The model under review builds one solid part; all positions refer to its coordinate system, in mm. A direction names the side the tool comes from. Coordinates: 2 decimals unless noted, no trailing zeros. Loops run counter-clockwise (first coordinate to the right, second up) from the corner with the lowest first, then second, coordinate; pieces in that order, holes last. Notation, with made-up numbers: (57.25, 61) - (91.25, 61) arc R28 ccw to (91.25, 96) - close; hole circle Ø4 at (7, 43). An arc over 180 degrees is marked (long way). Answer in a Markdown table with one row per item. Add a question column.
(1) Machinability: for faces 4 (the flat face through (21.61, 25.88, 11.01)), 5 (the cylindrical face through (24.116, 3.026, 5.916)), 6 (the flat face through (6.39, 25.88, 11.01)), which of the approach directions +Z, -Z, +X, -X, +Y, -Y give a long, thin tool a straight path to every point of the face, cutting with its end or side? Answer none if there is none.
(2) For line 1 along X through (y, z) = (5.25, 6); line 2 along Z through (x, y) = (-3.5, 5); line 3 along X through (y, z) = (1.5, 2), list the stretches that pass through material, from the lowest coordinate up.
(3) For P1, Ø1.5, axis at y = 23, z = 7.5, coming from the -X side; P2, Ø3.5, axis at x = -4, z = 5, coming from the +Y side; P3, Ø2, axis at x = 7, z = 11, coming from the -Y side, all flat-tipped, find the tip position at first contact; note any pin that passes through.
(4) We need section A-A on z = 6. Give the number of separate pieces and of enclosed holes in the cut face, plus the area to 3 significant figures.
(5) Mouldability with a two-part tool opening along X and no side actions: class faces 1 (the flat face through (14, 11, 12)), 2 (the flat face through (22.62, 26, 6)), 3 (the cylindrical face through (20.35, 26.03, 6.09)) as +X half, -X half, draft (parallel to the pull), parting line (faces both ways), or undercut.
(6) We need section B-B on y = 3. Write out the cut boundary in (x, z), plus the area to 3 significant figures.
(7) We need section C-C on x = 31.5. Write out the cut boundary in (y, z), plus the area to 3 significant figures.
(8) We need section D-D on y = 12.5. Write out the cut boundary in (x, z).
Autodesk Inventor part; units mm, degrees
ref_plane "Work Plane3" through (14, 0, 0) normal (-1, 0, 0) x (0, 0, 1)
ref_plane "YZ Plane" through (0, 0, 0) normal (1, 0, 0) x (0, 1, 0)
ref_plane "XZ Plane" through (0, 0, 0) normal (0, 1, 0) x (-1, 0, 0)
sketch "Sketch1" plane through (0, 0, 0) normal (0, 0, 1) x (1, 0, 0)
  line L0 (0, 0) -> (28, 0)
  line L1 (28, 0) -> (28, 28)
  line L2 (28, 28) -> (0, 28)
  line L3 (0, 28) -> (0, 0)
  circle A0 centre (7, 0) radius 4
  circle A1 centre (21, 0) radius 4 construction
  line L4 (21, 0) -> (23, 0) construction
  line L5 (20.5, 0) -> (21.5, 0) construction
  line L6 (20.5, -4) -> (21.5, -4)
  line L7 (21.5, 4) -> (20.5, 4)
  arc A2 (20.5, 4) -> (20.5, -4) centre (20.5, 0) ccw
  arc A3 (21.5, -4) -> (21.5, 4) centre (21.5, 0) ccw
  point P0 (3, 0)
  point P1 (11, 0)
  point P2 (17, 0)
  point P3 (25, 0)
  point P4 (21, 0)
  point P5 (16.5, 0)
  point P6 (25.5, 0)
  dimension "d0" = 28
  dimension "d1" = 28
  dimension "d2" = 8
  dimension "d3" = 8
  dimension "d4" = 14
  dimension "d5" = 7
  dimension "d6" = 7
  dimension "d41" = 1
extrude "Extrusion1" add sketch "Sketch1" along normal blind 12 contours L3 L2 L1 L0 A3 L7 A2 A0
chamfer "Chamfer1" distance 0.5 angle 45 4 edges at (3, 0, 6) (11, 0, 6) (16.5, 0, 6) (25.5, 0, 6)
sketch "Sketch2" plane through (0, 28, 0) normal (0, 1, 0) x (1, 0, 0)
  circle A0 centre (14, -6) radius 6.35
  line L0 (28, 0) -> (0, 0)
  line L1 (28, 0) -> (28, -12)
  point P0 (14, 0)
  point P1 (28, -6)
  point P2 (16.0791, 0)
  point P3 (11.9209, 0)
  dimension "d12" = 12.7
extrude "Extrusion2" cut sketch "Sketch2" against normal blind 4 contours A0 L0 picked at (13.6383, -8.0675)
fillet "Fillet1" radius 0.25 4 edges at (11.9209, 26, 0) (16.0791, 26, 0) (11.9209, 26, 12) (16.0791, 26, 12)
ref_plane "Work Plane3" through (14, 0, 0) normal (-1, 0, 0) x (0, 0, 1)
sketch "Sketch5" plane through (0, 0, 0) normal (0, -1, 0) x (1, 0, 0)
  circle A0 centre (-3.5, 6) radius 2
  circle A1 centre (-3.5, 6) radius 3.5
  circle A2 centre (-3.5, 6) radius 6
  line L0 (0, 12) -> (2.5, 12)
  line L1 (0, 0) -> (0, 12)
  line L2 (0, 0) -> (2.5, 0)
  line L3 (0, 0) -> (0, 12)
  line L4 (0, 0) -> (-5.9853, 0)
  line L5 (-5.9853, 0) -> (-7.7426, 1.7574)
  line L6 (0, 12) -> (-5.9853, 12)
  line L7 (-5.9853, 12) -> (-7.7426, 10.2426)
  line L8 (0, 0) -> (0, 12)
  line L9 (28, 0) -> (28, 12)
  line L10 (26, 0) -> (28, 0)
  line L11 (26, 12) -> (28, 12)
  line L12 (2.5, 12) -> (2.5, 0)
  line L13 (26, 0) -> (26, 12)
  dimension "d22" = 4
  dimension "d23" = 7
  dimension "d24" = 135
  dimension "d25" = 135
extrude "Extrusion3" add sketch "Sketch5" against normal blind 7 contours A0 | A1 | L1 A2 | L1 L4 A2 | A2 L6 L1 | L4 L5 A2 | A2 L7 L6 picked at (-7.4809, 9.2519)
sketch "Sketch6" plane through (2.5, 0, 0) normal (0, -1, 0) x (1, 0, 0)
  arc A0 (-10.2426, 10.2426) -> (-10.2426, 1.7574) centre (-6, 6) ccw
  point P0 (-2.5, 0)
hole "Hole1" at (-3.5, 0, 6) direction (0, 1, 0) diameter 4 end through all
mirror "Mirror2" about plane through (14, 0, 0) normal (-1, 0, 0) of "Extrusion3", "Hole1"
sketch "Sketch7" plane through (0, 0, 12) normal (0, 0, 1) x (1, 0, 0)
  line L0 (17.24, 24) -> (10.76, 24)
  line L1 (17.1173, 24) -> (17.24, 24)
  line L2 (17.1173, 24) -> (17.1173, 24)
  line L3 (17.24, 24) -> (17.1173, 24)
  line L4 (10.76, 24) -> (17.24, 24)
  line L5 (10.8827, 24) -> (10.76, 24)
  line L6 (10.8827, 24) -> (10.8827, 24)
  line L7 (10.76, 24) -> (10.8827, 24)
  line L8 (17.1173, 24) -> (20.35, 24)
  line L9 (7.65, 24) -> (10.8827, 24)
  line L10 (28, 28) -> (17.24, 28)
  line L11 (22.62, 28) -> (22.62, 24)
  line L12 (28, 7) -> (28, 28)
  line L13 (22.62, 24) -> (28, 7)
  line L14 (10.76, 28) -> (0, 28)
  line L15 (5.38, 28) -> (5.38, 24)
  line L16 (0, 28) -> (0, 7)
  line L17 (5.38, 24) -> (0, 7)
  line L18 (17.24, 24) -> (10.76, 24)
  point P0 (0, 0)
extrude "Extrusion4" cut sketch "Sketch7" against normal through all
chamfer "Chamfer2" distance 2 angle 45 8 edges at (22.62, 26, 12) (25.31, 15.5, 12) (22.62, 26, 0) (25.31, 15.5, 0) (2.69, 15.5, 12) (2.69, 15.5, 0) (5.38, 26, 0) (5.38, 26, 12)
equation "\"d1\" = MotorHeight"
equation "\"d5\" = d6"
equation "\"MotorHeight\" = MotorHeightBase"
properties part number "Magnet Mount"
Outcome:
| question | item | result |
|---|---|---|
| 1 | face 4 | +Z, +X, +Y |
| 1 | face 5 | +Z, -Z, -Y |
| 1 | face 6 | +Z, -X, +Y |
| 2 | line 1 | -9.5 to -5.5, -1.5 to 29.5, 33.5 to 37.5 |
| 2 | line 2 | 0 to 4, 8 to 12 |
| 2 | line 3 | -7.97 to 3.29, 10.71 to 16.79, 25.21 to 35.97 |
| 3 | P1 | x = 4.83 |
| 3 | P2 | y = 7 |
| 3 | P3 | y = 3.87 |
| 4 | separate pieces | 3 |
| 4 | enclosed holes | 0 |
| 4 | area | 621 mm² |
| 5 | face 1 | draft |
| 5 | face 2 | +X half |
| 5 | face 3 | undercut |
| 6 | outline | (-7.74, 1.76) - (-5.99, 0) - (4.35, 0) - (4.35, 12) - (-5.99, 12) - (-7.74, 10.24) arc R6 ccw to start; (9.65, 0) - (17.85, 0) - (17.85, 12) - (9.65, 12) - close; (24.15, 0) - (33.99, 0) - (35.74, 1.76) arc R6 ccw to (35.74, 10.24) - (33.99, 12) - (24.15, 12) - close; hole circle Ø4 at (-3.5, 6); hole circle Ø4 at (31.5, 6) |
| 6 | area | 372 mm² |
| 7 | outline | (0, 0) - (7, 0) - (7, 4) - (0, 4) - close; (0, 8) - (7, 8) - (7, 12) - (0, 12) - close |
| 7 | area | 56.0 mm² |
| 8 | outline | (1.74, 2) - (3.84, 0) - (24.16, 0) - (26.26, 2) - (26.26, 10) - (24.16, 12) - (3.84, 12) - (1.74, 10) - close |
